Input: part model. Units: mm. Frame: model coordinates. Face numbers are marked on the shaded views. A direction names the side the tool comes from. Round coordinates to 2 decimals unless told otherwise and drop trailing zeros. Loops run counter-clockwise (first coordinate to the right, second up) from the corner with the lowest first, then second, coordinate; pieces in that order, holes last. Notation, with made-up numbers: (26.25, 7) - (50.25, 7) arc R25 cw to (50.25, 33) - close; hole circle Ø8 at (70.25, -2.5). An arc over 180 degrees is marked (long way). One line per question, with ' | ' between items. Start each with the question number.
Item 1: Set-up query: the marked faces 1, 2, 3 and 4. Return all of +Z, -Z, +X, -X, +Y, -Y with unobstructed straight access to the full face (end or side cutting, diameter ignored); none if empty.
Item 2: First-contact query: pin 1 (3 mm diameter, centred on x = 7, z = 2.5, fed in from -Y); pin 2 (1 mm diameter, centred on x = 9.5, y = -1, fed in from +Z); pin 3 (0.7 mm diameter, centred on y = -1, z = 1, fed in from +X). Flat tips, straight axial feed; report the tip coordinate or a pass-through.
Item 3: Section A-A, the plane y = -1. Return loops of the section in (x, z), plus the area to 3 significant figures.
Item 4: Section C-C, the plane y = 0.5. Return loops of the section in (x, z).
Item 5: Section B-B, the plane x = 2.5. Return loops of the section in (y, z), plus the area to 3 significant figures.
Item 6: Section D-D, the plane x = 0.25. Return loops of the section in (y, z), plus the area to 3 significant figures.
Item 7: Material intervals for line 1 along X through (y, z) = (4.75, 5.5); line 2 along Y through (x, z) = (2.75, 2.6); line 3 along Y through (x, z) = (-1.5, 1.95), sorted ascending.
```python
from build123d import *

# Parameters (mm, degrees)
SKETCH1_W           = 11
SKETCH1_H           = 6
BOSS_EXTRUDE1_DEPTH = 5
SKETCH2_R           = 2.5
BOSS_EXTRUDE2_DEPTH = 3
SKETCH3_W           = 1.2
SKETCH3_H           = 0.6
BOSS_EXTRUDE3_DEPTH = 2.8


with BuildPart() as part:
    # Sketch1 → Boss-Extrude1 (new body)
    with BuildSketch(Plane(origin=(0, 0, 0), x_dir=(1, 0, 0), z_dir=(0, 1, 0))):
        with Locations((5.5, -3)):
            Rectangle(SKETCH1_W, SKETCH1_H)
    extrude(amount=BOSS_EXTRUDE1_DEPTH)

    # Sketch2 → Boss-Extrude2 (add)
    with BuildSketch(Plane.ZY):
        with Locations((3, 2.5)):
            Circle(SKETCH2_R)
    extrude(amount=BOSS_EXTRUDE2_DEPTH)

    # Sketch3 → Boss-Extrude3 (add)
    with BuildSketch(Plane(origin=(0, 0, 0), x_dir=(-1, 0, 0), z_dir=(0, -1, 0))):
        with Locations((-2.1, -0.8)):
            Rectangle(SKETCH3_W, SKETCH3_H)
        with Locations((-9.1, -0.8)):
            Rectangle(SKETCH3_W, SKETCH3_H)
        with Locations((-4.1, -5.2)):
            Rectangle(SKETCH3_W, SKETCH3_H)
    extrude(amount=BOSS_EXTRUDE3_DEPTH)


solid = part.part
```
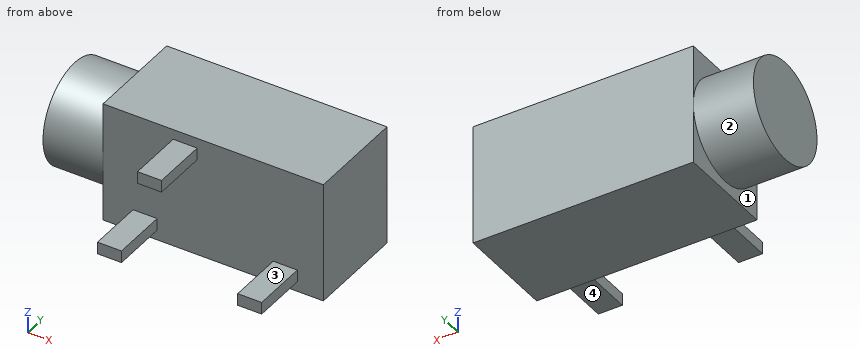
Return value:
1) face 1: -Z, -X | face 2: -X | face 3: +Z, +X, -X, -Y | face 4: -Z, +X, -X, -Y
2) pin 1: y = 0 | pin 2: z = 1.1 | pin 3: x = 9.7
3) outline: (1.5, 0.5) - (2.7, 0.5) - (2.7, 1.1) - (1.5, 1.1) - close; (3.5, 4.9) - (4.7, 4.9) - (4.7, 5.5) - (3.5, 5.5) - close; (8.5, 0.5) - (9.7, 0.5) - (9.7, 1.1) - (8.5, 1.1) - close | area: 2.16 mm2
4) outline: (-3, 1.5) - (0, 1.5) - (0, 0) - (11, 0) - (11, 6) - (0, 6) - (0, 4.5) - (-3, 4.5) - close
5) outline: (-2.8, 0.5) - (0, 0.5) - (0, 0) - (5, 0) - (5, 6) - (0, 6) - (0, 1.1) - (-2.8, 1.1) - close | area: 31.7 mm2
6) outline: (0, 0) - (5, 0) - (5, 6) - (0, 6) - close | area: 30.0 mm2
7) line 1: 0 to 11 | line 2: 0 to 5 | line 3: 0.23 to 4.77
